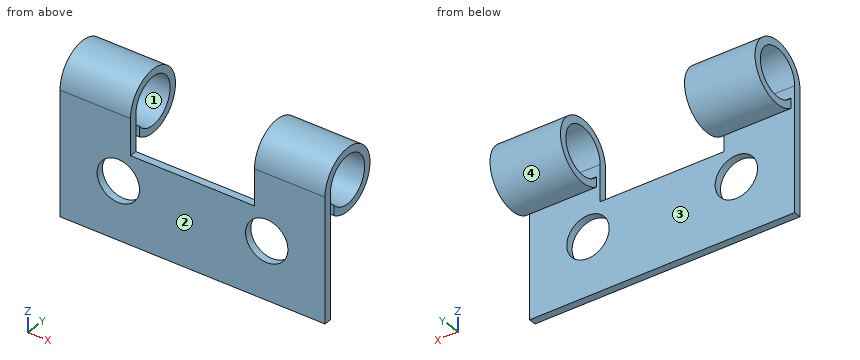
```python
from build123d import *

# Parameters (mm, degrees)
SALIENTE_EXTRUIR1_DEPTH    = 12.5
CORTAR_EXTRUIR1_REACH      = 21.475
CROQUIS5_R                 = 2
CORTAR_EXTRUIR2_DEPTH      = 20.475369059
CORTAR_EXTRUIR2_DEPTH_BACK = 20.475369059
CROQUIS6_W                 = 11.7
CROQUIS6_H                 = 6.4


with BuildPart() as part:
    # Croquis4 → Saliente-Extruir1 (new, symmetric)
    with BuildSketch(Plane(origin=(0, 0, 0), x_dir=(0, 0, -1), z_dir=(1, 0, 0))):
        with BuildLine():
            Line((14, 0), (14, 0.7))
            Line((14, 0.7), (2.25, 0.7))
            ThreePointArc((2.25, 0.7), (1.5, 5.071320344), (3.664213562, 1.2))
            Line((3.664213562, 1.2), (4.624868417, 1.2))
            ThreePointArc((4.624868417, 1.2), (0.91958653, 5.582964109), (2.25, 0))
            Line((2.25, 0), (14, 0))
        make_face()
    extrude(amount=SALIENTE_EXTRUIR1_DEPTH, both=True)

    # Croquis5 → Cortar-Extruir1 (cut, up to next)
    with BuildSketch(Plane(origin=(0, 0.7, 0), x_dir=(1, 0, 0), z_dir=(0, 1, 0)), mode=Mode.PRIVATE) as cortar_extruir1_sk1:
        with Locations(Location((7, 8.5, 0), (0, 0, 270))):
            Circle(CROQUIS5_R)
    cortar_extruir1_tool1 = extrude(cortar_extruir1_sk1.sketch, amount=-CORTAR_EXTRUIR1_REACH, mode=Mode.PRIVATE) & part.part
    # Croquis5 → Cortar-Extruir1 (cut, up to next)
    with BuildSketch(Plane(origin=(0, 0.7, 0), x_dir=(1, 0, 0), z_dir=(0, 1, 0)), mode=Mode.PRIVATE) as cortar_extruir1_sk2:
        with Locations(Location((-7, 8.5, 0), (0, 0, 270))):
            Circle(CROQUIS5_R)
    cortar_extruir1_tool2 = extrude(cortar_extruir1_sk2.sketch, amount=-CORTAR_EXTRUIR1_REACH, mode=Mode.PRIVATE) & part.part
    add(cortar_extruir1_tool1.solids().sort_by_distance((7, 0.7, -8.5))[0], mode=Mode.SUBTRACT)
    add(cortar_extruir1_tool2.solids().sort_by_distance((-7, 0.7, -8.5))[0], mode=Mode.SUBTRACT)

    # Croquis6 → Cortar-Extruir2 (cut, two sides: drawn at the far end of the back side and taken through both)
    with BuildSketch(Plane(origin=(0, 0.7, 0), x_dir=(1, 0, 0), z_dir=(0, 1, 0)).offset(-CORTAR_EXTRUIR2_DEPTH_BACK)):
        with Locations((0, 2.5)):
            Rectangle(CROQUIS6_W, CROQUIS6_H)
    extrude(amount=CORTAR_EXTRUIR2_DEPTH + CORTAR_EXTRUIR2_DEPTH_BACK, mode=Mode.SUBTRACT)


solid = part.part
```
Geometry check sheet. Reference: the model listing, model coordinates, mm. Face numbers are marked on the shaded views. A direction names the side the tool comes from. Coordinates: 2 decimals unless noted, no trailing zeros. Order: outer loops, then holes, each group sorted by start corner. A loop starts at its lowest first (then second) coordinate and runs counter-clockwise, first axis right, second up. Notation, with made-up numbers: M -29.5,1.25 L -6.5,1.25 A21 ccw -6.5,33.25 Z; hole C 46.25,-32.5 d9. An arc over 180 degrees is marked long. Answer as a JSON object with one key per item and string values.
Q1. Depth check by flat-ended pin: pin 1 Ø3.5 at (x, z) = (-7, -8.5) entering from -Y; pin 2 Ø3 at (x, y) = (9.5, 1) entering from +Z; pin 3 Ø1 at (x, z) = (-0.5, -7.5) entering from +Y; pin 4 Ø0.8 at (x, y) = (-2.5, 0.5) entering from +Z. Enter the tip coordinate at first touch or a pass-through.
Results are:
{"pin 1": "passes through", "pin 2": "stops at z = 0.67", "pin 3": "stops at y = 0.7", "pin 4": "stops at z = -5.7"}
Q2. Tool access check on the marked faces 3 and 4. Record the directions out of +Z, -Z, +X, -X, +Y, -Y that give a thin tool (end or side, any length) a straight path to the whole face; none if there is none.
Results are:
{"face 3": "-Z, +X, -X", "face 4": "+X, -X"}
Q3. Cross-section at D-D on y = 0.95. Record the cut outline in (x, z), and give its area (3 significant figures).
Results are:
{"outline": "M -12.5,-1.22 L -5.85,-1.22 L -5.85,-0.08 L -12.5,-0.08 Z; M 5.85,-1.22 L 12.5,-1.22 L 12.5,-0.08 L 5.85,-0.08 Z", "area": "15.1 mm²"}
Q4. Cross-section at C-C on z = -8.5. Record the cut outline in (x, y), and give its area (3 significant figures).
Results are:
{"outline": "M -12.5,0 L -9,0 L -9,0.7 L -12.5,0.7 Z; M -5,0 L 5,0 L 5,0.7 L -5,0.7 Z; M 9,0 L 12.5,0 L 12.5,0.7 L 9,0.7 Z", "area": "11.9 mm²"}
Q5. Cross-section at B-B on x = 7. Record the cut outline in (y, z).
Results are:
{"outline": "M 0,-14 L 0.7,-14 L 0.7,-10.5 L 0,-10.5 Z; M 0,-6.5 L 0.7,-6.5 L 0.7,-2.25 A2.25 cw long 1.2,-3.66 L 1.2,-4.62 A2.95 ccw long 0,-2.25 Z"}
Q6. Cross-section at A-A on y = 2.95. Record the cut outline in (x, z), and give its area (3 significant figures).
Results are:
{"outline": "M -12.5,-5.2 L -5.85,-5.2 L -5.85,-4.5 L -12.5,-4.5 Z; M -12.5,0 L -5.85,0 L -5.85,0.7 L -12.5,0.7 Z; M 5.85,-5.2 L 12.5,-5.2 L 12.5,-4.5 L 5.85,-4.5 Z; M 5.85,0 L 12.5,0 L 12.5,0.7 L 5.85,0.7 Z", "area": "18.6 mm²"}
Q7. Release check for a two-part mould opening along Y. For the marked faces 1 and 2 record: released by +Y, released by -Y, zero draft, split by the parting line, or undercut.
Results are:
{"face 1": "undercut", "face 2": "released by -Y"}
Q8. Scan lines: line 1 (X direction, y = 0.2, z = -8.5); line 2 (Z direction, x = 7.5, y = 2.95); line 3 (Y direction, x = -2.75, z = -8.5). Record each from-to range of solid material in increasing order.
Results are:
{"line 1": "x = -12.5 to -9, -5 to 5, 9 to 12.5", "line 2": "z = -5.2 to -4.5, 0 to 0.7", "line 3": "y = 0 to 0.7"}
